For this review, take the finished solid that the model builds, in its own axes (mm). Coordinates: 2 decimals unless noted, no trailing zeros. Loops run counter-clockwise (first coordinate to the right, second up) from the corner with the lowest first, then second, coordinate; pieces in that order, holes last. Notation, with made-up numbers: (45.5, 35.5) -> (67.5, 35.5) arc R22 cw to (67.5, 44.5) -> close; hole circle Ø10 at (7, 68). An arc over 180 degrees is marked (long way). One line per item, written item: value.
from build123d import *

# Parameters (mm, degrees)
SKETCH_1_W               = 70
SKETCH_1_H               = 70
SKETCH_1_R               = 30
EXTRUDE_1_DEPTH          = 3
SKETCH_2_R               = 2.1
CUT_EXTRUDE_1_DEPTH      = 10
PATTERN_CIRCULAR_1_COUNT = 4


with BuildPart() as part:
    # 草图1 → 凸台-拉伸1 (new body)
    with BuildSketch(Plane(origin=(0, 0, 0), x_dir=(1, 0, 0), z_dir=(0, 1, 0))):
        Rectangle(SKETCH_1_W, SKETCH_1_H)
        Circle(SKETCH_1_R, mode=Mode.SUBTRACT)
    extrude(amount=EXTRUDE_1_DEPTH)

    # 草图2 → 切除-拉伸1 (cut)
    with BuildSketch(Plane(origin=(0, 3, 0), x_dir=(1, 0, 0), z_dir=(0, 1, 0))):
        with Locations((27, 27)):
            Circle(SKETCH_2_R)
    cut_extrude_1 = extrude(amount=-CUT_EXTRUDE_1_DEPTH, mode=Mode.SUBTRACT)

    # 阵列(圆周)1: 切除-拉伸1 ×4 about axis
    pattern_circular_1_axis = Axis((0, 0, 0), (0, 1, 0))
    for i in range(1, PATTERN_CIRCULAR_1_COUNT):
        add(cut_extrude_1.rotate(pattern_circular_1_axis, i * 360 / PATTERN_CIRCULAR_1_COUNT), mode=Mode.SUBTRACT)


solid = part.part
1. Take a section at B-B, the plane z = -18. Give the boundary of the cut face in (x, y).
Return value:
outline: (-35, 0) -> (-24, 0) -> (-24, 3) -> (-35, 3) -> close; (24, 0) -> (35, 0) -> (35, 3) -> (24, 3) -> close
2. Take a section at A-A, the plane x = 0. Give the boundary of the cut face in (y, z).
Return value:
outline: (0, -35) -> (3, -35) -> (3, -30) -> (0, -30) -> close; (0, 30) -> (3, 30) -> (3, 35) -> (0, 35) -> close
3. The part is to be moulded in two halves that separate along Z. For faces 1 (the flat face through (-35, 1, 0)), 2 (the flat face through (0, 1, 35)), 3 (the cylindrical face through (25.137, 1.521, 27.969)), 4 (the flat face through (0, 1, -35)), say which applies: pulls with the +Z half, pulls with the -Z half, needs draft (parallel to the pull), parting line crosses it, or undercut.
Return value:
face 1: needs draft
face 2: pulls with the +Z half
face 3: undercut
face 4: pulls with the -Z half
4. Take a section at D-D, the plane x = -27. Give the boundary of the cut face in (y, z).
Return value:
outline: (0, -35) -> (3, -35) -> (3, -29.1) -> (0, -29.1) -> close; (0, -24.9) -> (3, -24.9) -> (3, -13.08) -> (0, -13.08) -> close; (0, 13.08) -> (3, 13.08) -> (3, 24.9) -> (0, 24.9) -> close; (0, 29.1) -> (3, 29.1) -> (3, 35) -> (0, 35) -> close
5. To check wall thickness, follow probe 1 along X at (y, z) = (1, -27); probe 2 along X at (y, z) = (2.2, 0). State the ranges of each line that lie inside material, in increasing order. Write a range as from..to.
Return value:
probe 1: x = -35..-29.1, -24.9..-13.08, 13.08..24.9, 29.1..35
probe 2: x = -35..-30, 30..35
6. Take a section at C-C, the plane y = 1.95. Give the boundary of the cut face in (x, z).
Return value:
outline: (-35, -35) -> (35, -35) -> (35, 35) -> (-35, 35) -> close; hole circle Ø60 at (0, 0); hole circle Ø4.2 at (-27, -27); hole circle Ø4.2 at (-27, 27); hole circle Ø4.2 at (27, -27); hole circle Ø4.2 at (27, 27)
